Design review of the part shown in the three views and the two pictorial views. Dimensions are in mm from the part's minimum x, y and z. Coordinates: 2 decimals unless noted, no trailing zeros. Write each loop counter-clockwise with the first axis right and the second up, starting at its lowest first coordinate (ties: lowest second). Pieces come first, ordered by that corner, then holes. Notation, with made-up numbers: (33.5, 52) -> (56.5, 52) arc R26 ccw to (56.5, 86) -> close; hole circle Ø10 at (59.5, 55). An arc over 180 degrees is marked (long way). Write each question's results on one line, items separated by ' | '.
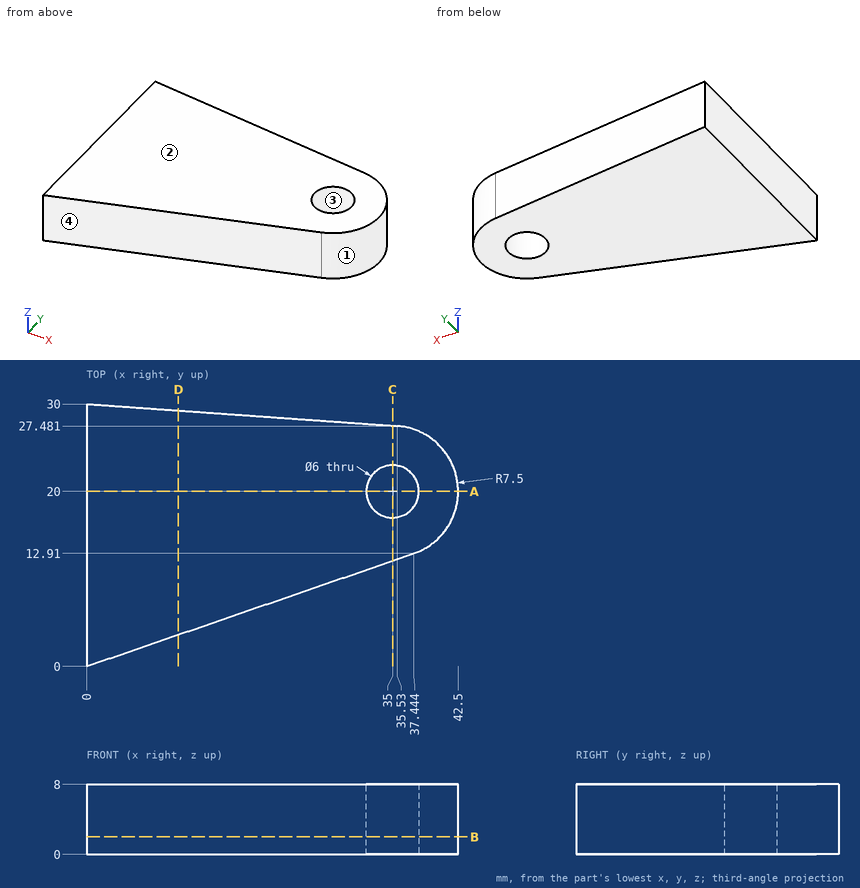
Q1. Add section B-B (z = 2). Write out the cut boundary in (x, y) (1 decimal), plus the area to 3 significant figures.
Solution:
outline: (0, 0) -> (37.4, 12.9) arc R7.5 ccw to (35.5, 27.5) -> (0, 30) -> close; hole circle Ø6 at (35, 20) | area: 856 mm²
Q2. Draft analysis for pull direction Y (two halves, no side actions). For the marked faces 1, 2, 3 and 4, state which applies: pulls with the +Y half, pulls with the -Y half, needs draft (parallel to the pull), parting line crosses it, or undercut.
Solution:
face 1: parting line crosses it | face 2: needs draft | face 3: undercut | face 4: pulls with the -Y half
Q3. Add section C-C (x = 35). Write out the cut boundary in (y, z).
Solution:
outline: (12.07, 0) -> (17, 0) -> (17, 8) -> (12.07, 8) -> close; (23, 0) -> (27.52, 0) -> (27.52, 8) -> (23, 8) -> close
Q4. Clearance check with flat-ended pins moving along their axes: P1, Ø3, axis at x = 26, y = 8.5, coming from the +Z side; P2, Ø3, axis at x = 38, z = 2, coming from the +Y side; P3, Ø2, axis at y = 13.5, z = 1.5, coming from the +X side; P4, Ø4, axis at x = 24.5, z = 5.5, coming from the +Y side (1 decimal). State where each tip first meets the part, or that it passes through.
Solution:
P1: z = 8 | P2: y = 27.35 | P3: x = 40.1 | P4: y = 28.4
Q5. For line 1 (Y direction, x = 35, z = 3); line 2 (Y direction, x = 4, z = 4.5) (1 decimal); line 3 (Y direction, x = 22, z = 4) (1 decimal), list the stretches that pass through material, from the lowest coordinate up. Write a range as from..to.
Solution:
line 1: 12.07..17, 23..27.52 | line 2: 1.4..29.7 | line 3: 7.6..28.4
Q6. Add section A-A (y = 20). Write out the cut boundary in (x, z).
Solution:
outline: (0, 0) -> (32, 0) -> (32, 8) -> (0, 8) -> close; (38, 0) -> (42.5, 0) -> (42.5, 8) -> (38, 8) -> close
Q7. Add section D-D (x = 10.5). Write out the cut boundary in (y, z) (1 decimal), plus the area to 3 significant figures.
Solution:
outline: (3.6, 0) -> (29.3, 0) -> (29.3, 8) -> (3.6, 8) -> close | area: 205 mm²
